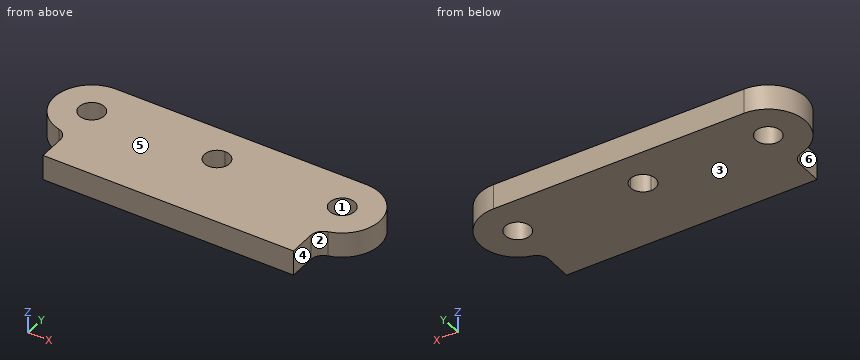
from build123d import *

# Parameters (mm, degrees)
F0_R     = 5
F1_DEPTH = 10


with BuildPart() as f1:
    # F0 (on Top) → F1 (new body)
    with BuildSketch(Plane.XY):
        with BuildLine():
            Line((0, 15), (-50, 15))
            ThreePointArc((-50, 15), (-64.880445, 1.890064), (-53.75, -14.523688))
            ThreePointArc((-53.75, -14.523688), (-51.047153, -16.303055), (-50, -19.364917))
            Line((-50, -19.364917), (-50, -30))
            Line((-50, -30), (0, -30))
            Line((0, -30), (0, -5))
            ThreePointArc((0, -5), (-5, 0), (0, 5))
            Line((0, 5), (0, 15))
        make_face()
        with Locations((-50, 0)):
            Circle(F0_R, mode=Mode.SUBTRACT)
        with BuildLine():
            Line((50, 15), (0, 15))
            Line((0, 15), (0, 5))
            ThreePointArc((0, 5), (3.535534, 3.535534), (5, 0))
            ThreePointArc((5, 0), (3.535534, -3.535534), (0, -5))
            Line((0, -5), (0, -30))
            Line((0, -30), (50, -30))
            Line((50, -30), (50, -19.364917))
            ThreePointArc((50, -19.364917), (51.047153, -16.303055), (53.75, -14.523688))
            ThreePointArc((53.75, -14.523688), (64.880445, 1.890064), (50, 15))
        make_face()
        with BuildLine():
            ThreePointArc((55, 0), (50, -5), (45, 0))
            ThreePointArc((45, 0), (50, 5), (55, 0))
        make_face(mode=Mode.SUBTRACT)
    extrude(amount=F1_DEPTH)


solid = f1.part
Part model, mm, in its own coordinate system. Face numbers are marked on the shaded views. A direction names the side the tool comes from. Round coordinates to 2 decimals unless told otherwise and drop trailing zeros. Write each loop counter-clockwise with the first axis right and the second up, starting at its lowest first coordinate (ties: lowest second). Pieces come first, ordered by that corner, then holes. Notation, with made-up numbers: M 48.5,-38.5 L 79.5,-38.5 A18 cw 79.5,-30.5 Z; hole C -0.75,-33 d2. An arc over 180 degrees is marked long. Return JSON: item names as keys, results as strings. Group by question number.
(1) Which spindle directions (+Z, -Z, +X, -X, +Y, -Y) get a long thin tool onto all of the face, cutting with end or side? Do the marked faces 4, 5 and 6. Say none if no direction does.
(2) Saw through at C-C on y = 2. Write the cut outline in (x, z), then the cut area to 3 significant figures.
(3) Drill centre lines: probe 1 along X at (y, z) = (-20, 3.5); probe 2 along X at (y, z) = (1.5, 7); probe 3 along X at (y, z) = (3.5, 6.25). Where is each one in solid material? Low to high.
(4) Saw through at B-B on z = 3.25. Write the cut outline in (x, y), then the cut area to 3 significant figures.
(5) Pin check, flat tips, straight feed: pin 1 Ø4 at (y, z) = (9, 2.5) entering from +X; pin 2 Ø1 at (y, z) = (-1, 6) entering from +X; pin 3 Ø6 at (x, y) = (50, 0) entering from +Z. Stop position of each tip, or through.
(6) Saw through at A-A on y = -3. Write the cut outline in (x, z), then the cut area to 3 significant figures.
(7) Two-plate mould, pull along Y, no slides. Class the marked faces 1, 2 and 3: +Y half, -Y half, draft (parallel to the pull), parting line (faces both ways), or undercut.
(8) Saw through at D-D on y = -17. Write the cut outline in (x, z), then the cut area to 3 significant figures.
Returned:
{
 "1": {"face 4": "+Z, -Z, +X, -Y", "face 5": "+Z, +X, -X, +Y, -Y", "face 6": "+Z, -Z, -X, -Y"},
 "2": {"outline": "M -64.87,0 L -54.58,0 L -54.58,10 L -64.87,10 Z; M -45.42,0 L -4.58,0 L -4.58,10 L -45.42,10 Z; M 4.58,0 L 45.42,0 L 45.42,10 L 4.58,10 Z; M 54.58,0 L 64.87,0 L 64.87,10 L 54.58,10 Z", "area": "1,020 mm²"},
 "3": {"probe 1": "-50 to 50", "probe 2": "-64.92 to -54.77, -45.23 to -4.77, 4.77 to 45.23, 54.77 to 64.92", "probe 3": "-64.59 to -53.57, -46.43 to -3.57, 3.57 to 46.43, 53.57 to 64.59"},
 "4": {"outline": "M -53.75,-14.52 A5 cw -50,-19.36 L -50,-30 L 50,-30 L 50,-19.36 A5 cw 53.75,-14.52 A15 ccw 50,15 L -50,15 A15 ccw Z; hole C -50,0 d10; hole C 0,0 d10; hole C 50,0 d10", "area": "4,980 mm²"},
 "5": {"pin 1": "x = 63.27", "pin 2": "x = 64.99", "pin 3": "through"},
 "6": {"outline": "M -64.7,0 L -54,0 L -54,10 L -64.7,10 Z; M -46,0 L -4,0 L -4,10 L -46,10 Z; M 4,0 L 46,0 L 46,10 L 4,10 Z; M 54,0 L 64.7,0 L 64.7,10 L 54,10 Z", "area": "1,050 mm²"},
 "7": {"face 1": "undercut", "face 2": "-Y half", "face 3": "draft"},
 "8": {"outline": "M -50.59,0 L 50.59,0 L 50.59,10 L -50.59,10 Z", "area": "1,010 mm²"}
}
